from build123d import *

# Parameters (mm, degrees)
SKETCH1_R           = 2.6
BOSS_EXTRUDE1_DEPTH = 20
BOSS_EXTRUDE2_DEPTH = 180
CUT_EXTRUDE1_DEPTH  = 192.378764777


with BuildPart() as part:
    # Sketch1 → Boss-Extrude1 (new body)
    with BuildSketch(Plane(origin=(0, 0, 0), x_dir=(1, 0, 0), z_dir=(0, 1, 0))):
        with BuildLine():
            Line((10, 0), (-10, 0))
            ThreePointArc((-10, 0), (-4.705844869, 30.024645745), (10.538067282, 56.427876097))
            Line((10.538067282, 56.427876097), (25.858956145, 43.572123903))
            ThreePointArc((25.858956145, 43.572123903), (14.088007547, 23.184242879), (10, 0))
        make_face()
        with Locations(Location((0.645465629, 10, 0), (0, 0, 270))):
            Circle(SKETCH1_R, mode=Mode.SUBTRACT)
        with Locations(Location((4.691081339, 26.604444312, 0), (0, 0, 270))):
            Circle(SKETCH1_R, mode=Mode.SUBTRACT)
        with Locations(Location((12.265090975, 41.92465826, 0), (0, 0, 270))):
            Circle(SKETCH1_R, mode=Mode.SUBTRACT)
    extrude(amount=BOSS_EXTRUDE1_DEPTH)

    # Sketch3 → Cut-Extrude1 (cut, through all)
    with BuildSketch(Plane(origin=(0, 20, 0), x_dir=(1, 0, 0), z_dir=(0, 1, 0))):
        with BuildLine():
            Line((25.858956145, 43.572123903), (10.538067282, 56.427876097))
            ThreePointArc((10.538067282, 56.427876097), (-4.705844869, 30.024645745), (-10, 0))
            Line((-10, 0), (10, 0))
            ThreePointArc((10, 0), (14.088007547, 23.184242879), (25.858956145, 43.572123903))
        make_face()
    extrude(amount=-CUT_EXTRUDE1_DEPTH, mode=Mode.SUBTRACT)


with BuildPart() as body_2:
    # Sketch2 → Boss-Extrude2 (new body)
    with BuildSketch(Plane(origin=(0, 20, 0), x_dir=(1, 0, 0), z_dir=(0, 1, 0))):
        with BuildLine():
            Line((6.707845067, 59.641814145), (10.538067282, 56.427876097))
            ThreePointArc((10.538067282, 56.427876097), (-4.705844869, 30.024645745), (-10, 0))
            Line((-10, 0), (-15, 0))
            ThreePointArc((-15, 0), (-9.404307973, 31.734746462), (6.707845067, 59.641814145))
        make_face()
    extrude(amount=BOSS_EXTRUDE2_DEPTH)


solid = body_2.part
Can you work these out from the model? Positions are in its coordinate system, mm. Give positions to 0.01 mm unless a question says otherwise; leave off trailing zeros. Loops run counter-clockwise (first coordinate to the right, second up) from the corner with the lowest first, then second, coordinate; pieces in that order, holes last. Notation, with made-up numbers: (26.5, 54) - (51.5, 54) arc R19 ccw to (51.5, 66) - close; hole circle Ø10 at (53.5, 13.25). An arc over 180 degrees is marked (long way). One line per item, written item: value.
(1) I need wall thicknesses on line 1 along X through (y, z) = (123.5, -49); line 2 along X through (y, z) = (115, -46); line 3 along Z through (x, y) = (6.5, 80.5). Which ranges of each line are inside material? Lowest first, please.
Verdict:
line 1: -1.01 to 4.95
line 2: -2.79 to 3.02
line 3: -59.39 to -51.23
(2) If we section it at B-B, the plane z = -11: List the corners of the cut face in (x, y) for me.
Verdict:
outline: (-14.35, 20) - (-9.31, 20) - (-9.31, 200) - (-14.35, 200) - close
(3) If we section it at A-A, the plane y = 138.5: List the corners of the cut face in (x, z) for me, plus the area to 3 significant figures.
Verdict:
outline: (-15, 0) arc R92.79 ccw to (6.71, -59.64) - (10.54, -56.43) arc R87.79 cw to (-10, 0) - close
area: 315 mm^2
(4) I'm going to push flat-ended pins straight in: pin 1 (5 mm diameter, centred on x = -0.5, y = 149, fed in from +Z); pin 2 (5 mm diameter, centred on y = 101.5, z = -9, fed in from -X); pin 3 (8 mm diameter, centred on y = 63, z = -15, fed in from +X). Where does each tip first touch, or does it pass through?
Verdict:
pin 1: z = -34.35
pin 2: x = -14.77
pin 3: x = -7.92
